Autodesk Inventor part; units mm, degrees
ref_plane "YZ Plane" through (0, 0, 0) normal (1, 0, 0) x (0, 1, 0)
ref_plane "XZ Plane" through (0, 0, 0) normal (0, 1, 0) x (-1, 0, 0)
ref_plane "XY Plane" through (0, 0, 0) normal (0, 0, 1) x (1, 0, 0)
sketch "Náčrt1" plane through (0, 0, 0) normal (0, 0, 1) x (1, 0, 0)
  circle A0 centre (13.025, 0) radius 8.05
  circle A1 centre (-13.025, 0) radius 8.05
  line L0 (22.5, 0) -> (22.5, 10)
  line L1 (22.5, 10) -> (-22.5, 10)
  line L2 (-22.5, 10) -> (-22.5, -20)
  line L3 (-22.5, -20) -> (22.5, -20)
  line L4 (22.5, -20) -> (22.5, 0)
  point P0 (0, 0)
  point P1 (0, 0)
  dimension "d2" = 16.1
  dimension "d5" = 10
  dimension "d6" = 30
  dimension "d18" = 16.1
extrude "Vysunutí1" add sketch "Náčrt1" along normal blind 5
sketch "Náčrt2" plane through (0, 0, 0) normal (0, 0, -1) x (-1, 0, 0)
  line L0 (-22.5, -20) -> (-22.5, 10)
  line L1 (-22.5, -20) -> (22.5, -20)
  line L2 (22.5, -20) -> (22.5, -15)
  line L3 (22.5, -15) -> (-22.5, -15)
  line L4 (-22.5, -15) -> (-22.5, -20)
  point P0 (0, 0)
  dimension "d9" = 45
  dimension "d10" = 5
extrude "Vysunutí2" add sketch "Náčrt2" along normal blind 25
sketch "Náčrt3" plane through (-22.5, -15, 0) normal (0, 1, 0) x (1, 0, 0)
  circle A0 centre (40, 22) radius 2
  line L0 (45, 0) -> (45, 25)
  line L1 (0, 25) -> (45, 25)
  line L2 (22.5, 25) -> (22.5, 18.3064)
  circle A1 centre (5, 22) radius 2
  point P0 (22.5, 0)
  dimension "d13" = 4
  dimension "d14" = 5
  dimension "d15" = 3
extrude "Vysunutí3" cut sketch "Náčrt3" against normal blind 25
fillet "Zaoblení1" radius 5 4 edges at (-22.5, 10, 2.5) (22.5, 10, 2.5) (22.5, -17.5, -25) (-22.5, -17.5, -25)
fillet "Zaoblení2" radius 5 1 edges at (0, -15, 0)
properties part number "distance sensor"
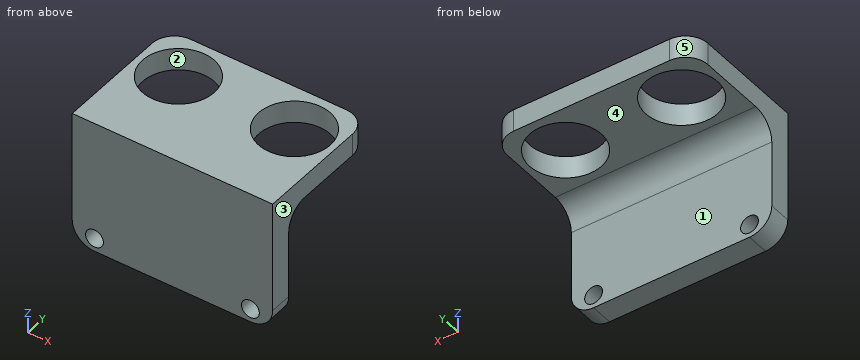
Geometry check sheet. Reference: the model listing, model coordinates, mm. Face numbers are marked on the shaded views. A direction names the side the tool comes from. Give positions to 0.01 mm unless a question says otherwise; leave off trailing zeros. Order: outer loops, then holes, each group sorted by start corner. A loop starts at its lowest first (then second) coordinate and runs counter-clockwise, first axis right, second up.
1. Section check B-B, the plane x = -6.5. Enter the section's corners in (y, z), and give its area (3 significant figures).
2. Section check A-A, the plane y = 0. Enter the section's corners in (x, z) (3 decimals), and give its area (3 significant figures).
3. Thickness scan on L1, parallel to X at y = 0.25, z = 0.25; L2, parallel to X at y = -16.4, z = -22; L3, parallel to Z at x = 17.5, y = -17.05. Record the ranges inside material, lowest first.
4. Access from +Z, -Z, +X, -X, +Y, -Y to the whole of each face (thin tool, end or side, straight path). Record for the marked faces 4 and 5.
5. Release check for a two-part mould opening along Y. For the marked faces 1, 2 and 3 record: pulls with the +Y half, pulls with the -Y half, needs draft (parallel to the pull), parting line crosses it, or undercut.
6. Gauge pin test, flat ends, axial feed: pin 1 Ø2 at (x, z) = (15, -7.5) entering from +Y; pin 2 Ø16 at (x, y) = (0.5, 1.5) entering from -Z; pin 3 Ø16 at (x, z) = (-2, -10.5) entering from +Y. Record the tip position at first contact, or that the pin passes through.
7. Section check D-D, the plane x = -16. Enter the section's corners in (y, z).
8. Section check C-C, the plane z = -23. Enter the section's corners in (x, y), and give its area (3 significant figures).
Values follow:
1. outline: (-20, -25) - (-15, -25) - (-15, -5) arc R5 cw to (-10, 0) - (-4.71, 0) - (-4.71, 5) - (-20, 5) - close; (4.71, 0) - (10, 0) - (10, 5) - (4.71, 5) - close
1. area: 233 mm2
2. outline: (-22.5, 0) - (-21.075, 0) - (-21.075, 5) - (-22.5, 5) - close; (-4.975, 0) - (4.975, 0) - (4.975, 5) - (-4.975, 5) - close; (21.075, 0) - (22.5, 0) - (22.5, 5) - (21.075, 5) - close
2. area: 64.0 mm2
3. L1: x = -22.5 to -21.07, -4.98 to 4.98, 21.07 to 22.5
3. L2: x = -22.08 to -19.5, -15.5 to 15.5, 19.5 to 22.08
3. L3: z = -25 to -24, -20 to 5
4. face 4: -Z, +X, -X, +Y
4. face 5: +Z, -Z, -X, +Y
5. face 1: pulls with the +Y half
5. face 2: undercut
5. face 3: needs draft
6. pin 1: stops at y = -15
6. pin 2: stops at z = 0
6. pin 3: stops at y = -14.33
7. outline: (-20, -25) - (-15, -25) - (-15, -23.32) - (-20, -23.32) - close; (-20, -20.68) - (-15, -20.68) - (-15, -5) arc R5 cw to (-10, 0) - (-7.48, 0) - (-7.48, 5) - (-20, 5) - close; (7.48, 0) - (10, 0) - (10, 5) - (7.48, 5) - close
8. outline: (-21.5, -20) - (-19.23, -20) - (-19.23, -15) - (-21.5, -15) - close; (-15.77, -20) - (15.77, -20) - (15.77, -15) - (-15.77, -15) - close; (19.23, -20) - (21.5, -20) - (21.5, -15) - (19.23, -15) - close
8. area: 180 mm2
